from build123d import *

# Parameters (mm, degrees)
SKETCH_1_W          = 25
SKETCH_1_H          = 50
EXTRUDE_1_DEPTH     = 1.5
SKETCH_2_R          = 1.5
SKETCH_2_R_2        = 2
SKETCH_2_R_3        = 0.4
CUT_EXTRUDE_1_DEPTH = 56.921820428


with BuildPart() as part:
    # Эскиз1 → Бобышка-Вытянуть1 (new body)
    with BuildSketch(Plane(origin=(0, 0, 0), x_dir=(1, 0, 0), z_dir=(0, 1, 0))):
        with Locations((12.5, 25)):
            Rectangle(SKETCH_1_W, SKETCH_1_H)
    extrude(amount=EXTRUDE_1_DEPTH)

    # Эскиз2 → Вырез-Вытянуть1 (cut, through all)
    with BuildSketch(Plane(origin=(0, 1.5, 0), x_dir=(1, 0, 0), z_dir=(0, 1, 0))):
        with Locations((25, 25)):
            Circle(SKETCH_2_R)
        with Locations((0, 25)):
            Circle(SKETCH_2_R)
        with Locations((25, 0)):
            Circle(SKETCH_2_R_2)
        Circle(SKETCH_2_R_2)
        with Locations((0, 50)):
            Circle(SKETCH_2_R_2)
        with Locations((25, 50)):
            Circle(SKETCH_2_R_2)
        with Locations(Location((3.5, 40, 0), (0, 0, 270))):
            Circle(SKETCH_2_R_3)
        with Locations(Location((3.5, 37.46, 0), (0, 0, 270))):
            Circle(SKETCH_2_R_3)
        with Locations(Location((3.5, 34.92, 0), (0, 0, 270))):
            Circle(SKETCH_2_R_3)
        with Locations(Location((3.5, 14.42, 0), (0, 0, 270))):
            Circle(SKETCH_2_R_3)
        with Locations(Location((3.5, 11.88, 0), (0, 0, 270))):
            Circle(SKETCH_2_R_3)
        with Locations(Location((3.5, 9.34, 0), (0, 0, 270))):
            Circle(SKETCH_2_R_3)
        with Locations(Location((21.5, 40, 0), (0, 0, 270))):
            Circle(SKETCH_2_R_3)
        with Locations(Location((21.5, 37.46, 0), (0, 0, 270))):
            Circle(SKETCH_2_R_3)
        with Locations(Location((21.5, 34.92, 0), (0, 0, 270))):
            Circle(SKETCH_2_R_3)
        with Locations(Location((21.5, 14.42, 0), (0, 0, 270))):
            Circle(SKETCH_2_R_3)
        with Locations(Location((21.5, 11.88, 0), (0, 0, 270))):
            Circle(SKETCH_2_R_3)
        with Locations(Location((21.5, 9.34, 0), (0, 0, 270))):
            Circle(SKETCH_2_R_3)
    extrude(amount=-CUT_EXTRUDE_1_DEPTH, mode=Mode.SUBTRACT)


solid = part.part
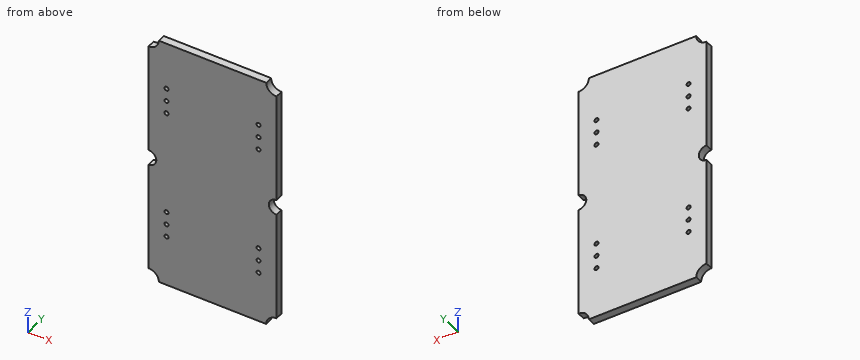
Geometry: final body of the model. Coordinates: model frame, mm. Coordinates: 2 decimals unless noted, no trailing zeros. Loops run counter-clockwise (first coordinate to the right, second up) from the corner with the lowest first, then second, coordinate; pieces in that order, holes last. Notation, with made-up numbers: (35, 10) - (45, 10) arc R16 ccw to (45, 18) - close; hole circle Ø1 at (-26.5, 28.5). An arc over 180 degrees is marked (long way). Put each result on its own line as item: value. Start each with the question number.
Q1. Line query: line 1 (X direction, y = 0.9, z = -9.34). Output: solid intervals per line, ascending.
Q2. Cut plane A-A, the plane y = 0.9. Give the number of separate pieces and of enclosed holes in the cut face, and give its area (3 significant figures).
Q3. Cut plane B-B, the plane z = -25. Return loops of the section in (x, y).
Filled sheet:
1. line 1: 0 to 3.1, 3.9 to 21.1, 21.9 to 25
2. separate pieces: 1
2. enclosed holes: 12
2. area: 1,220 mm²
3. outline: (1.5, 0) - (23.5, 0) - (23.5, 1.5) - (1.5, 1.5) - close
